Verification items for the finished model (mm, model axes). Face numbers are marked on the shaded views. A direction names the side the tool comes from. Round coordinates to 2 decimals unless told otherwise and drop trailing zeros. Write each loop counter-clockwise with the first axis right and the second up, starting at its lowest first coordinate (ties: lowest second). Pieces come first, ordered by that corner, then holes. Notation, with made-up numbers: (-21.75, 40.5) - (-12.75, 40.5) arc R12 cw to (-12.75, 50.5) - close; hole circle Ø1 at (65.5, -6). An arc over 180 degrees is marked (long way). Answer as a JSON object with one key per item and string values.
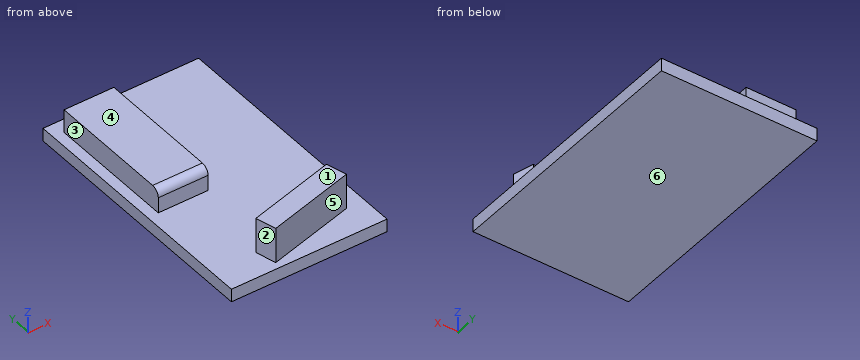
```python
from build123d import *

# Parameters (mm, degrees)
F0_W     = 300
F0_H     = 500
F1_DEPTH = 25
F2_W     = 96
F2_H     = 250
F3_DEPTH = 45
F5_DEPTH = 68
F6_R     = 15


with BuildPart() as f1:
    # F0 (on Top) → F1 (new body)
    with BuildSketch(Plane.XY):
        with Locations((-100.745436, 14.865042)):
            Rectangle(F0_W, F0_H)
    extrude(amount=F1_DEPTH)

    # F2 (on face) → F3 (join)
    with BuildSketch(Plane.XY.offset(25)):
        with Locations((-182.168748, 112.275026)):
            Rectangle(F2_W, F2_H)
    extrude(amount=F3_DEPTH)

    # F4 (on face) → F5 (join)
    with BuildSketch(Plane.XY.offset(25)):
        Polygon((3.368272, -137.631641), (-165.668748, -182.924974), (-155.315986, -221.562007), (13.721034, -176.268674), align=None)
    extrude(amount=F5_DEPTH)

    # F6
    f6_edges = [f1.edges().sort_by_distance(p)[0] for p in [
        (-182.168748, -12.724974, 70),
    ]]
    fillet(f6_edges, radius=F6_R)


solid = f1.part
```
1. Material ranges on probe 1 along Z at (x, y) = (11, 175.5); probe 2 along Z at (x, y) = (-177.5, 28.5); probe 3 along X at (y, z) = (209, 39.5), recorded low to high. Write a range as from..to.
Completed:
{"probe 1": "z = 0..25", "probe 2": "z = 0..70", "probe 3": "x = -230.17..-134.17"}
2. Cross-section at C-C (x = -185.5). Record the boundary of the cut face in (y, z), plus the area to 3 significant figures.
Completed:
{"outline": "(-235.13, 0) - (264.87, 0) - (264.87, 25) - (237.28, 25) - (237.28, 70) - (2.28, 70) arc R15 ccw to (-12.72, 55) - (-12.72, 25) - (-235.13, 25) - close", "area": "23,700 mm^2"}
3. Cross-section at D-D (z = 63). Record the boundary of the cut face in (x, y).
Completed:
{"outline": "(-230.17, -10.41) - (-134.17, -10.41) - (-134.17, 237.28) - (-230.17, 237.28) - close; (-165.67, -182.92) - (-155.32, -221.56) - (13.72, -176.27) - (3.37, -137.63) - close"}
4. Cross-section at B-B (y = 27.5). Record the boundary of the cut face in (x, z), plus the area to 3 significant figures.
Completed:
{"outline": "(-250.75, 0) - (49.25, 0) - (49.25, 25) - (-134.17, 25) - (-134.17, 70) - (-230.17, 70) - (-230.17, 25) - (-250.75, 25) - close", "area": "11,800 mm^2"}
5. Mould release check, pull along Y, two halves, no side actions. Record for the marked faces 5 and 6: released by +Y, released by -Y, zero draft, split by the parting line, or undercut.
Completed:
{"face 5": "released by -Y", "face 6": "zero draft"}
6. Go/stop test with flat-tipped pins: pin 1 (22.5 mm diameter, centred on x = -183, z = 44, fed in from +Y) (3 decimals); pin 2 (15 mm diameter, centred on x = -182.5, z = 44.5, fed in from -Y) (3 decimals); pin 3 (12 mm diameter, centred on y = 131, z = 51, fed in from +X). Record where each tip stops, or that it passes through.
Completed:
{"pin 1": "stops at y = 237.275", "pin 2": "stops at y = -12.725", "pin 3": "stops at x = -134.17"}
7. Cross-section at A-A (z = 34). Record the boundary of the cut face in (x, y), plus the area to 3 significant figures.
Completed:
{"outline": "(-230.17, -12.72) - (-134.17, -12.72) - (-134.17, 237.28) - (-230.17, 237.28) - close; (-165.67, -182.92) - (-155.32, -221.56) - (13.72, -176.27) - (3.37, -137.63) - close", "area": "31,000 mm^2"}
8. Access from +Z, -Z, +X, -X, +Y, -Y to the whole of each face (thin tool, end or side, straight path). Record for the marked faces 1, 2, 3 and 4.
Completed:
{"face 1": "+Z, +X, -X, +Y, -Y", "face 2": "+Z, -X, -Y", "face 3": "+Z, -X, +Y, -Y", "face 4": "+Z, +X, -X, +Y"}
